Part model, mm, in its own coordinate system. A direction names the side the tool comes from. Round coordinates to 2 decimals unless told otherwise and drop trailing zeros. Loops run counter-clockwise (first coordinate to the right, second up) from the corner with the lowest first, then second, coordinate; pieces in that order, holes last. Notation, with made-up numbers: M 32,-24 L 62,-24 A11 cw 62,-17 Z; hole C 37,-26 d2. An arc over 180 degrees is marked long. Answer as CSV lines item,"result". Start each with the question number.
Item 1: Wall check: line 1 (Y direction, x = 8.5, z = 17.25); line 2 (Z direction, x = -1, y = -20); line 3 (X direction, y = -9.5, z = 16). Give the ranges that are in metal, low to high.
Item 2: Drop flat-ended pins along their axis: pin 1 Ø12 at (y, z) = (5, 12.5) entering from -X; pin 2 Ø10 at (x, y) = (5, -1) entering from +Z. Give the stop position or say it passes through.
Item 3: Band-saw the part on B-B (z = 13.5). Give the cut face in (x, y).
Item 4: Band-saw the part on A-A (x = 8.25). Give the cut face in (y, z).
Item 5: Which spindle directions (+Z, -Z, +X, -X, +Y, -Y) get a long thin tool onto all of the face, cutting with end or side? Do faces 1 (the flat face through (-2.791, -4.4, 4.8)), 2 (the flat face through (7, -11, 5)). Say none if no direction does.
```python
from build123d import *

# Parameters (mm, degrees)
SKETCH1_W           = 55
SKETCH1_H           = 25
BOSS_EXTRUDE1_DEPTH = 5
BOSS_EXTRUDE2_DEPTH = 15


with BuildPart() as part:
    # Sketch1 → Boss-Extrude1 (new body)
    with BuildSketch(Plane(origin=(0, 0, 0), x_dir=(0, 1, 0), z_dir=(0, 0, 1))):
        with Locations((-8.366983373, -9.709026128)):
            Rectangle(SKETCH1_W, SKETCH1_H)
    extrude(amount=BOSS_EXTRUDE1_DEPTH)

    # Sketch3 → Boss-Extrude2 (add)
    with BuildSketch(Plane.XY.offset(5)):
        Polygon((-2.790973872, 14.133016627), (-2.790973872, 19.133016627), (22.209026128, 19.133016627), (22.209026128, -35.866983373), (17.209026128, -35.866983373), (17.209026128, 14.133016627), align=None)
    extrude(amount=BOSS_EXTRUDE2_DEPTH)


solid = part.part
```
Answer block:
1,line 1,"y = 14.13 to 19.13"
1,line 2,"z = 0 to 5"
1,line 3,"x = 17.21 to 22.21"
2,pin 1,"stops at x = 17.21"
2,pin 2,"stops at z = 5"
3,outline,"M -2.79,14.13 L 17.21,14.13 L 17.21,-35.87 L 22.21,-35.87 L 22.21,19.13 L -2.79,19.13 Z"
4,outline,"M -35.87,0 L 19.13,0 L 19.13,20 L 14.13,20 L 14.13,5 L -35.87,5 Z"
5,face 1,"+Z, -Z, -X, +Y, -Y"
5,face 2,"+Z, -X, -Y"
